from build123d import *

# Parameters (mm, degrees)
SKETCH1_R           = 3
BOSS_EXTRUDE1_DEPTH = 8.9
CHAMFER1_SIZE       = 0.2
SKETCH2_R           = 3
BOSS_EXTRUDE2_DEPTH = 10
SKETCH3_R           = 1.75
BOSS_EXTRUDE3_DEPTH = 0.2
BOSS_EXTRUDE4_DEPTH = 2.5


with BuildPart() as part:
    # Sketch1 → Boss-Extrude1 (new body)
    with BuildSketch(Plane.XY):
        Circle(SKETCH1_R)
    extrude(amount=BOSS_EXTRUDE1_DEPTH)

    # Chamfer1
    chamfer1_edges = [part.edges().sort_by_distance(p)[0] for p in [
        (-3, 0, 0),
        (-3, 0, 8.9),
    ]]
    chamfer(chamfer1_edges, length=CHAMFER1_SIZE)

    # Sketch2 → Boss-Extrude2 (add)
    with BuildSketch(Plane.XY.offset(8.9)):
        Circle(SKETCH2_R)
    extrude(amount=BOSS_EXTRUDE2_DEPTH)

    # Sketch3 → Boss-Extrude3 (add)
    with BuildSketch(Plane.XY.offset(18.9)):
        Circle(SKETCH3_R)
    extrude(amount=BOSS_EXTRUDE3_DEPTH)

    # Sketch5 → Boss-Extrude4 (add)
    with BuildSketch(Plane.XY.offset(19.1)):
        with BuildLine():
            Line((0, 0.49), (0.848704896, 0.49))
            ThreePointArc((0.848704896, 0.49), (0, -0.98), (-0.848704896, 0.49))
            Line((-0.848704896, 0.49), (0, 0.49))
        make_face()
    extrude(amount=BOSS_EXTRUDE4_DEPTH)


solid = part.part
The model under review builds one solid part; all positions refer to its coordinate system, in mm. A direction names the side the tool comes from. Coordinates: 2 decimals unless noted, no trailing zeros. Loops run counter-clockwise (first coordinate to the right, second up) from the corner with the lowest first, then second, coordinate; pieces in that order, holes last. Notation, with made-up numbers: M 37,-37.5 L 93,-37.5 A31 ccw 93,-9.5 Z; hole C 41,82.5 d8. An arc over 180 degrees is marked long. Put each result on its own line as item: value. Start each with the question number.
Q1. Add section A-A (x = 0). Write out the cut boundary in (y, z).
Q2. Clearance check with flat-ended pins moving along their axes: pin 1 (1.9 mm diameter, centred on x = 0.5, z = 21, fed in from +Y); pin 2 (2 mm diameter, centred on x = -1.5, z = 11.5, fed in from +Y); pin 3 (1.5 mm diameter, centred on y = -2, z = 11, fed in from +X). State where each tip first meets the part, or that it passes through.
Q3. For faces 1 (the flat face through (0, -2, 18.9)), 2 (the flat face through (0, 0.49, 20)), 3 (the cylindrical face through (-3, 0, 4)), list the 3-axis set-ups (+Z, -Z, +X, -X, +Y, -Y) from which the entire face can be reached by the end or side of a thin tool; tool diameter is ignored.
Q4. Wall thickness on line 1 (X direction, y = 0.1, z = 12.5); line 2 (Z direction, x = 2.7, y = 0.35); line 3 (Z direction, x = -0.9, y = -1.45): over which ranges is each line inside the solid? List them lowest first.
Q5. Add section B-B (y = 0). Write out the cut boundary in (x, z), and give its area (3 significant figures).
Q6. Add section C-C (z = 7.75). Write out the cut boundary in (x, y), and give its area (3 significant figures).
Answers:
1. outline: M -3,0.2 L -2.8,0 L 2.8,0 L 3,0.2 L 3,8.7 L 2.8,8.9 L 3,8.9 L 3,18.9 L 1.75,18.9 L 1.75,19.1 L 0.49,19.1 L 0.49,21.6 L -0.98,21.6 L -0.98,19.1 L -1.75,19.1 L -1.75,18.9 L -3,18.9 L -3,8.9 L -2.8,8.9 L -3,8.7 Z
2. pin 1: stops at y = 0.49
2. pin 2: stops at y = 2.96
2. pin 3: stops at x = 2.73
3. face 1: +Z
3. face 2: +Z, +X, -X, +Y
3. face 3: +Z, -Z
4. line 1: x = -3 to 3
4. line 2: z = 0 to 18.9
4. line 3: z = 0 to 19.1
5. outline: M -3,0.2 L -2.8,0 L 2.8,0 L 3,0.2 L 3,8.7 L 2.8,8.9 L 3,8.9 L 3,18.9 L 1.75,18.9 L 1.75,19.1 L 0.98,19.1 L 0.98,21.6 L -0.98,21.6 L -0.98,19.1 L -1.75,19.1 L -1.75,18.9 L -3,18.9 L -3,8.9 L -2.8,8.9 L -3,8.7 Z
5. area: 119 mm^2
6. outline: C 0,0 d6
6. area: 28.3 mm^2
